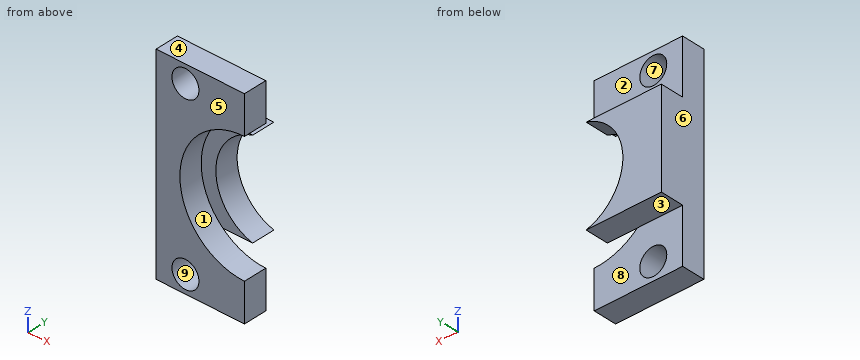
Autodesk Inventor part; units mm, degrees
ref_plane "YZ Plane" through (0, 0, 0) normal (1, 0, 0) x (0, 1, 0)
ref_plane "XZ Plane" through (0, 0, 0) normal (0, 1, 0) x (-1, 0, 0)
ref_plane "XY Plane" through (0, 0, 0) normal (0, 0, 1) x (1, 0, 0)
sketch "Sketch1" plane through (0, 0, 0) normal (0, 1, 0) x (-1, 0, 0)
  line L0 (-0.3136, 9.3425) -> (-7.8416, 9.3425)
  line L1 (-7.8416, -8.1575) -> (-0.3136, -8.1575)
  line L2 (-0.3136, -8.1575) -> (-0.3136, 9.3425)
  circle A0 centre (-2.8136, 7.8425) radius 1.15
  circle A1 centre (-2.8136, -6.6575) radius 1.15
  arc A2 (-7.8416, -3.6575) -> (-7.8416, 4.8425) centre (-7.8416, 0.5925) ccw
  line L3 (-7.8416, 9.3425) -> (-7.8416, 4.8425)
  line L4 (-7.8416, -3.6575) -> (-7.8416, -8.1575)
  point P0 (0, 0)
  point P1 (0, 0)
  dimension "d0" = 17.5
  dimension "d1" = 2.5
  dimension "d2" = 2.5
  dimension "d3" = 1.5
  dimension "d4" = 1.5
  dimension "d5" = 2.3
  dimension "d6" = 2.3
  dimension "d7" = 8.5
  dimension "d8" = 7.528
  dimension "d9" = 8.75
extrude "Extrusion1" add sketch "Sketch1" along normal blind 4
sketch "Sketch3" plane through (0, 0, 0) normal (0, -1, 0) x (1, 0, 0)
  circle A0 centre (7.8416, 0.5925) radius 5.5
  line L0 (7.8416, 9.3425) -> (7.8416, 4.8425)
  line L1 (7.8416, -8.1575) -> (0.3136, -8.1575)
  point P0 (0, 0)
  dimension "d12" = 11
  dimension "d13" = 0
  dimension "d14" = 8.75
extrude "Extrusion2" cut sketch "Sketch3" against normal blind 2
sketch "Sketch4" plane through (0, 4, 0) normal (0, 1, 0) x (1, 0, 0)
  line L0 (7.8416, -9.3425) -> (0.3136, -9.3425)
  line L1 (0.3136, -9.3425) -> (0.3136, -4.6925)
  line L2 (0.3136, -4.6925) -> (7.8416, -4.6925)
  line L3 (7.8416, -4.6925) -> (7.8416, -9.3425)
  line L4 (7.8416, 3.6575) -> (7.8416, 8.1575)
  line L5 (0.3136, 8.1575) -> (0.3136, -9.3425)
  line L6 (7.8416, 8.1575) -> (0.3136, 8.1575)
  line L7 (0.3136, 8.1575) -> (0.3136, 3.5075)
  line L8 (0.3136, 3.5075) -> (7.8416, 3.5075)
  line L9 (7.8416, 3.5075) -> (7.8416, 8.1575)
  point P0 (0, 0)
  dimension "d17" = 4.65
  dimension "d18" = 4.65
  dimension "d23" = 0
extrude "Extrusion3" cut sketch "Sketch4" against normal blind 2 contours L0 L1 L2 L3
extrude "Extrusion4" cut sketch "Sketch4" against normal blind 2 contours L5 L6 L4 L9 L8
properties part number "UCover_PWR"
Geometry check sheet. Reference: the model listing, model coordinates, mm. Face numbers are marked on the shaded views. A direction names the side the tool comes from. Coordinates: 2 decimals unless noted, no trailing zeros. Loops run counter-clockwise (first coordinate to the right, second up) from the corner with the lowest first, then second, coordinate; pieces in that order, holes last.
Item 1: Sectioned sample at D-D, the plane x = 1.25. Record the boundary of the cut face in (y, z).
Item 2: Sectioned sample at C-C, the plane y = 1.45. Record the boundary of the cut face in (x, z), then the cut area to 3 significant figures.
Item 3: Release check for a two-part mould opening along X. For the marked faces 6, 7, 8 and 9 record: released by +X, released by -X, zero draft, split by the parting line, or undercut.
Item 4: Access from +Z, -Z, +X, -X, +Y, -Y to the whole of each face (thin tool, end or side, straight path). Record for the marked faces 1, 2, 3, 4 and 5.
Item 5: Sectioned sample at A-A, the plane x = 5.75. Record the boundary of the cut face in (y, z).
Item 6: Thickness scan on line 1 (Z direction, x = 7.75, y = 1.4); line 2 (Z direction, x = 3.5, y = 1.9); line 3 (Z direction, x = 3.75, y = 1.75). Record the ranges inside material, lowest first.
Item 7: Go/stop test with flat-tipped pins: pin 1 Ø0.6 at (x, y) = (3, 3) entering from -Z; pin 2 Ø3.5 at (x, z) = (3.5, 6.5) entering from +Y; pin 3 Ø1.6 at (x, y) = (2.5, 3.5) entering from +Z. Record where each tip stops, or that it passes through.
Item 8: Sectioned sample at B-B, the plane z = 8. Record the boundary of the cut face in (x, y), then the cut area to 3 significant figures.
Check result:
1. outline: (0, -8.16) - (2, -8.16) - (2, -3.51) - (4, -3.51) - (4, 4.69) - (2, 4.69) - (2, 9.34) - (0, 9.34) - close
2. outline: (0.31, -8.16) - (7.84, -8.16) - (7.84, -4.91) arc R5.5 cw to (7.84, 6.09) - (7.84, 9.34) - (0.31, 9.34) - close; hole circle Ø2.3 at (2.81, -6.66); hole circle Ø2.3 at (2.81, 7.84)
2. area: 75.9 mm2
3. face 6: released by -X
3. face 7: undercut
3. face 8: zero draft
3. face 9: undercut
4. face 1: +X, -Y
4. face 2: +Z, +X, -X, +Y
4. face 3: -Z, +X, -X, +Y
4. face 4: +Z, +X, -X, +Y, -Y
4. face 5: +Z, -Z, +X, -X, -Y
5. outline: (0, -8.16) - (2, -8.16) - (2, -4.49) - (0, -4.49) - close; (0, 5.68) - (2, 5.68) - (2, 9.34) - (0, 9.34) - close; (2, -3.51) - (4, -3.51) - (4, -3.11) - (2, -3.11) - close; (2, 4.29) - (4, 4.29) - (4, 4.69) - (2, 4.69) - close
6. line 1: z = -8.16 to -4.91, 6.09 to 9.34
6. line 2: z = -8.16 to -7.58, -5.73 to -2.78, 3.97 to 6.92, 8.77 to 9.34
6. line 3: z = -8.16 to -7.33, -5.99 to -3.08, 4.27 to 7.17, 8.51 to 9.34
7. pin 1: stops at z = -3.51
7. pin 2: stops at y = 2
7. pin 3: stops at z = 4.69
8. outline: (0.31, 0) - (1.67, 0) - (1.67, 2) - (0.31, 2) - close; (3.95, 0) - (7.84, 0) - (7.84, 2) - (3.95, 2) - close
8. area: 10.5 mm2
